Geometry: see drawing. Coordinates: mm, zero at the bounding-box minimum. A direction names the side the tool comes from. Round coordinates to 2 decimals unless told otherwise and drop trailing zeros. Loops run counter-clockwise (first coordinate to the right, second up) from the corner with the lowest first, then second, coordinate; pieces in that order, holes last. Notation, with made-up numbers: (6, 33.5) - (65, 33.5) arc R27 cw to (65, 56.5) - close; hole circle Ø10 at (-5, 56). An arc over 180 degrees is marked (long way). Use CSV: the item, a comma, the result in double quotes. Start each with the question number.
1. Cut plane C-C (y = 497). Return loops of the section in (x, z).
2. Material intervals for probe 1 along Y at (x, z) = (11.5, 123); probe 2 along Z at (x, y) = (69.5, 631); probe 3 along X at (y, z) = (1443, 148), sorted ascending. Write a range as from..to.
3. Cut plane B-B (x = 49). Return loops of the section in (y, z), and give its area (3 significant figures).
4. Access query for the marked faces 4 and 5. Directions: +Z, -Z, +X, -X, +Y, -Y. A direction counts if a zero-diameter tool reaches every point of the face in a straight line with its end or side. Return the directions, or none.
5. Cut plane A-A (z = 146). Return loops of the section in (x, y), and give its area (3 significant figures).
6. Pull-direction query (Y, two-part tool) for the marked faces 1, 2 and 3; classes: +Y half, -Y half, draft (parallel to the pull), parting line (faces both ways), or undercut.
7. Pin query (flat end, axial travel): P1, Ø5, axis at y = 935, z = 166.5, coming from the +X side; P2, Ø4, axis at x = 58, y = 858.5, coming from the +Z side. Return the tip coordinate at first contact, or that it passes through.
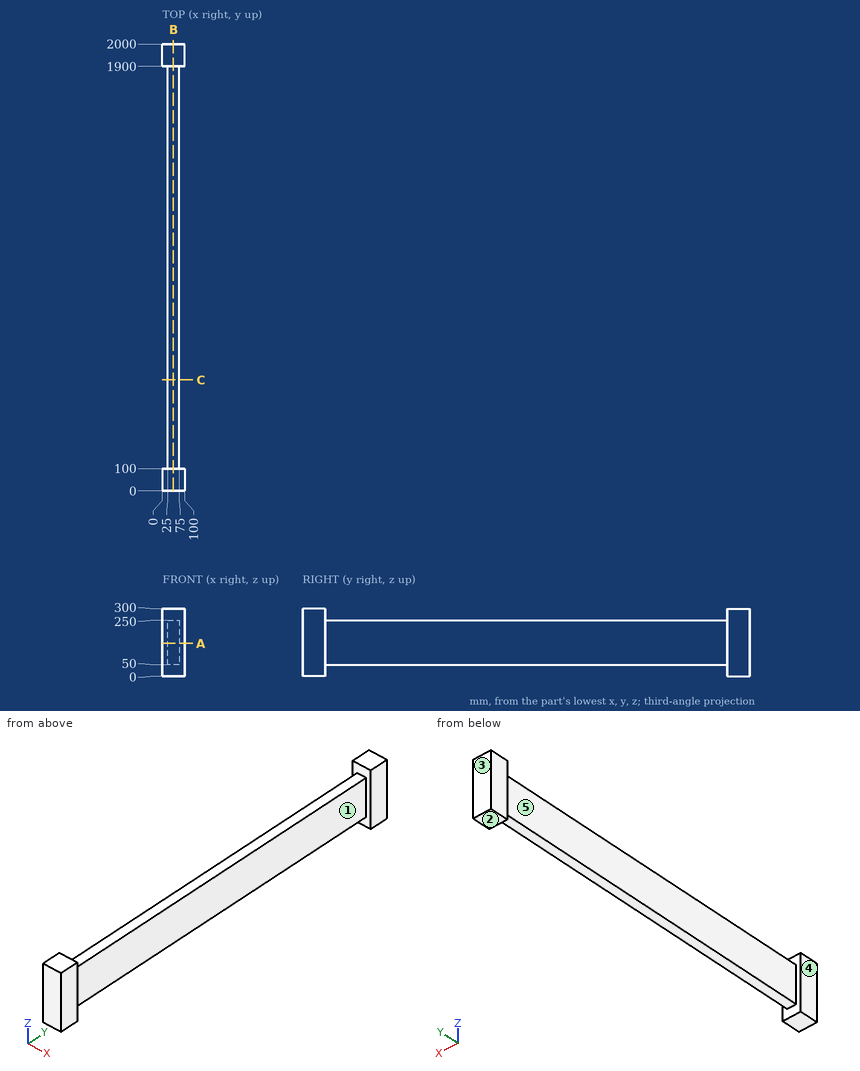
Established:
1,outline,"(25, 50) - (75, 50) - (75, 250) - (25, 250) - close"
2,probe 1,"y = 0..100, 1900..2000"
2,probe 2,"z = 50..250"
2,probe 3,"x = 25..75"
3,outline,"(0, 0) - (100, 0) - (100, 50) - (1900, 50) - (1900, 0) - (2000, 0) - (2000, 300) - (1900, 300) - (1900, 250) - (100, 250) - (100, 300) - (0, 300) - close"
3,area,"420,000 mm2"
4,face 4,"+Z, -Z, -X, +Y, -Y"
4,face 5,"+Z, -Z, -X"
5,outline,"(0, 0) - (100, 0) - (100, 100) - (75, 100) - (75, 1900) - (100, 1900) - (100, 2000) - (0, 2000) - (0, 1900) - (25, 1900) - (25, 100) - (0, 100) - close"
5,area,"110,000 mm2"
6,face 1,"undercut"
6,face 2,"draft"
6,face 3,"+Y half"
7,P1,"stops at x = 75"
7,P2,"stops at z = 250"
